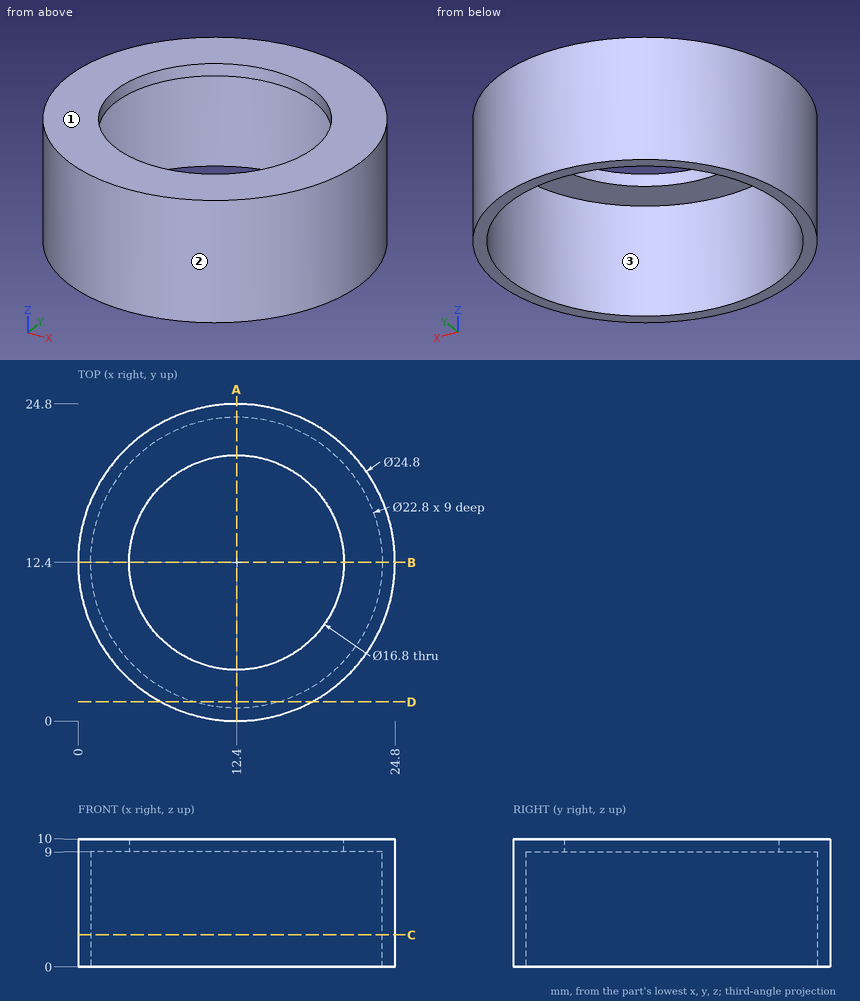
Could you check a few things on this drawing? It's one solid part, dimensions in mm from its lowest x, y, z. Coordinates: 2 decimals unless noted, no trailing zeros. Write each loop counter-clockwise with the first axis right and the second up, starting at its lowest first coordinate (ties: lowest second). Pieces come first, ordered by that corner, then holes. Notation, with made-up numbers: (-26.75, 16.5) - (30.25, 16.5) arc R26 ccw to (30.25, 35.5) - close; hole circle Ø5 at (11, 39.25). An arc over 180 degrees is marked (long way). Return JSON: item names as keys, results as strings. Group by question number.
Item 1: If we section it at C-C (z = 2.5): Write out the boundary of the cut face in (x, y).
Item 2: I'm going to push flat-ended pins straight in: pin 1 Ø1.5 at (y, z) = (9, 6.5) entering from +X; pin 2 Ø1.5 at (x, y) = (18.5, 5.5) entering from -Z; pin 3 Ø1.5 at (y, z) = (11, 8) entering from +X. Where does each tip first touch, or does it pass through?
Item 3: If we section it at A-A (x = 12.4): Write out the boundary of the cut face in (y, z), then the cut area to 3 significant figures.
Item 4: Please list where these lines run through material, in increasing order: probe 1 along Y at (x, z) = (12.4, 4.5); probe 2 along Y at (x, z) = (12.4, 9.6); probe 3 along Z at (x, y) = (22.5, 8.25).
Item 5: If we section it at D-D (y = 1.5): Write out the boundary of the cut face in (x, z), then the cut area to 3 significant figures.
Item 6: We'd pull the mould along X, two halves only. Please class the marked faces 1, 2 and 3: pulls with the +X half, pulls with the -X half, needs draft (parallel to the pull), parting line crosses it, or undercut.
Return value:
{
 "1": {"outline": "circle Ø24.8 at (12.4, 12.4); hole circle Ø22.8 at (12.4, 12.4)"},
 "2": {"pin 1": "stops at x = 24.51", "pin 2": "stops at z = 9", "pin 3": "stops at x = 24.78"},
 "3": {"outline": "(0, 0) - (1, 0) - (1, 9) - (4, 9) - (4, 10) - (0, 10) - close; (20.8, 9) - (23.8, 9) - (23.8, 0) - (24.8, 0) - (24.8, 10) - (20.8, 10) - close", "area": "26.0 mm^2"},
 "4": {"probe 1": "y = 0 to 1, 23.8 to 24.8", "probe 2": "y = 0 to 4, 20.8 to 24.8", "probe 3": "z = 9 to 10"},
 "5": {"outline": "(6.49, 0) - (9.06, 0) - (9.06, 9) - (15.74, 9) - (15.74, 0) - (18.31, 0) - (18.31, 10) - (6.49, 10) - close", "area": "58.1 mm^2"},
 "6": {"face 1": "needs draft", "face 2": "parting line crosses it", "face 3": "undercut"}
}
